CAD build for the part. Positions are in the model's coordinates, mm. A direction names the side the tool comes from. Coordinates: 2 decimals unless noted, no trailing zeros. Loops run counter-clockwise (first coordinate to the right, second up) from the corner with the lowest first, then second, coordinate; pieces in that order, holes last. Notation, with made-up numbers: (87.5, -19.5) -> (125.5, -19.5) arc R27 cw to (125.5, 13.5) -> close; hole circle Ø11 at (-28.75, 18). An arc over 180 degrees is marked (long way). Write each question's results on one line, items separated by ' | '.
```python
from build123d import *

# Parameters (mm, degrees)
SKETCH3_R                = 15
CUT_EXTRUDE1_DEPTH       = 10
SKETCH4_W                = 17
SKETCH4_H                = 15
CUT_EXTRUDE2_DEPTH       = 32.819805153
SKETCH4_4_W              = 27
SKETCH4_4_H              = 25
SKETCH4_4_W_2            = 17
SKETCH4_4_H_2            = 15
EXTRUDE_THIN2_DEPTH      = 160
SKETCH5_W                = 10
SKETCH5_H                = 60
BOSS_EXTRUDE1_DEPTH      = 3
FILLET1_R                = 4
BOSS_EXTRUDE5_DEPTH      = 9
BOSS_EXTRUDE5_DEPTH_BACK = 5
SKETCH6_W                = 36
SKETCH6_H                = 40
CUT_EXTRUDE4_DEPTH       = 17
CUT_EXTRUDE4_DEPTH_BACK  = 160
SKETCH2_3_R              = 14.5
CUT_EXTRUDE5_DEPTH       = 170.068033643
CUT_EXTRUDE5_DEPTH_BACK  = 170.068033643
SKETCH8_W                = 9
SKETCH8_H                = 8
FILLET2_R                = 34
FILLET3_R                = 34
BOSS_EXTRUDE6_DEPTH      = 20


with BuildPart() as part:
    # Extrude-Thin1: read off the stored shape, not the designer's step
    # Extrude-Thin1 outline → Extrude-Thin1 (revolve)
    with BuildSketch(Plane.XZ):
        Polygon((17.5, 20), (0, 20), (0, 17), (14.5, 17), (14.5, 3), (0, 3), (0, 0), (17.5, 0), align=None)
    revolve(axis=Axis((0, 0, 0), (0, 0, 1)))

    # Sketch3 → Cut-Extrude1 (cut)
    with BuildSketch(Plane(origin=(0, 0, 0), x_dir=(-1, 0, 0), z_dir=(0, 0, -1))):
        Circle(SKETCH3_R)
    extrude(amount=-CUT_EXTRUDE1_DEPTH, mode=Mode.SUBTRACT)

    # Sketch4 → Cut-Extrude2 (cut, through all)
    with BuildSketch(Plane(origin=(0, 0, 0), x_dir=(0, 0, -1), z_dir=(1, 0, 0))):
        with Locations((-8.5, 0)):
            Rectangle(SKETCH4_W, SKETCH4_H)
    extrude(amount=CUT_EXTRUDE2_DEPTH, mode=Mode.SUBTRACT)

    # Sketch4<4> → Extrude-Thin2 (add)
    with BuildSketch(Plane(origin=(0, 0, 0), x_dir=(0, 0, -1), z_dir=(1, 0, 0))):
        with Locations((-8.5, 0)):
            Rectangle(SKETCH4_4_W, SKETCH4_4_H)
        with Locations((-8.5, 0)):
            Rectangle(SKETCH4_4_W_2, SKETCH4_4_H_2, mode=Mode.SUBTRACT)
    extrude(amount=EXTRUDE_THIN2_DEPTH)

    # Sketch5 → Boss-Extrude1 (add)
    with BuildSketch(Plane(origin=(0, 0, 0), x_dir=(-1, 0, 0), z_dir=(0, 0, -1))):
        Rectangle(SKETCH5_W, SKETCH5_H)
    extrude(amount=-BOSS_EXTRUDE1_DEPTH)

    # Fillet1
    fillet1_edges = [part.edges().sort_by_distance(p)[0] for p in [
        (-5, 30, 1.5),
        (5, -30, 1.5),
        (-5, -30, 1.5),
        (5, 30, 1.5),
    ]]
    fillet(fillet1_edges, radius=FILLET1_R)

    # Sketch6 → Boss-Extrude5 (add, two sides: drawn at the far end of the back side and taken through both)
    with BuildSketch(Plane.ZY.offset(17.5).offset(-BOSS_EXTRUDE5_DEPTH_BACK)):
        with Locations((2, 0)):
            Rectangle(SKETCH6_W, SKETCH6_H)
    extrude(amount=BOSS_EXTRUDE5_DEPTH + BOSS_EXTRUDE5_DEPTH_BACK)

    # Sketch2<3> → Cut-Extrude4 (cut, two sides: drawn at the far end of the back side and taken through both)
    with BuildSketch(Plane.XY.offset(-CUT_EXTRUDE4_DEPTH_BACK)):
        with Locations(Location((0, 0, 0), (0, 0, 149.549685979))):
            Circle(SKETCH2_3_R)
    extrude(amount=CUT_EXTRUDE4_DEPTH + CUT_EXTRUDE4_DEPTH_BACK, mode=Mode.SUBTRACT)

    # Sketch8 → Cut-Extrude5 (cut, two sides: drawn at the far end of the back side and taken through both)
    with BuildSketch(Plane.XZ.offset(20).offset(-CUT_EXTRUDE5_DEPTH_BACK)):
        with Locations((-17, -4)):
            Rectangle(SKETCH8_W, SKETCH8_H)
    extrude(amount=CUT_EXTRUDE5_DEPTH + CUT_EXTRUDE5_DEPTH_BACK, mode=Mode.SUBTRACT)

    # Fillet2
    # the kernel refuses this fillet: 34 mm, written as the material it adds along each edge
    with BuildSketch(Plane(origin=(-12.5, -12.247448714, 0), x_dir=(0.923034160497627, -0.3847179987399096, 0), z_dir=(0, 0, 1))) as fillet2_piece_1:
        with BuildLine():
            CenterArc((26.914388587, -31.306789136), FILLET2_R, 112.958457005, 21.780491129)
            Line((2.982546016, -7.155869668), (2.503909164, -6.672851279))
            ThreePointArc((2.503909164, -6.672851279), (0.863609779, -3.839543073), (-0.627663229, -0.261608239))
            Line((-0.627663229, -0.261608239), (0.26524325, 0.626135783))
            ThreePointArc((0.26524325, 0.626135783), (6.826113047, -0.706211474), (13.386982845, 0.626135783))
            Line((13.386982845, 0.626135783), (13.652226095, 0))
        make_face()
    extrude(amount=20)
    with BuildSketch(Plane(origin=(-12.5, 12.247448714, 0), x_dir=(0, 1, 0), z_dir=(0, 0, 1))) as fillet2_piece_2:
        with BuildLine():
            CenterArc((39.251685543, -12.798614811), FILLET2_R, 157.887286265, 21.780491129)
            Line((5.252257101, -12.601471052), (4.572268533, -12.597528177))
            ThreePointArc((4.572268533, -12.597528177), (3.277985866, -6.029043261), (-0.475900864, -0.485714286))
            Line((-0.475900864, -0.485714286), (0, 0.68))
            ThreePointArc((0, 0.68), (3.876275643, 0.68), (7.122568601, 0.255972296))
            Line((7.122568601, 0.255972296), (7.752551286, 0))
        make_face()
    extrude(amount=20)

    # Fillet3
    # the kernel refuses this fillet: 34 mm, written as the material it adds along each edge
    with BuildSketch(Plane(origin=(0, 12.5, 20), x_dir=(-1, 0, 0), z_dir=(0, -1, 0))) as fillet3_piece_1:
        with BuildLine():
            CenterArc((11.489125293, -34), FILLET3_R, 90, 19.749922796)
            Line((0, -2), (0, 0))
            Line((0, 0), (11.489125293, 0))
        make_face()
    extrude(amount=25)

    # Sketch9 → Boss-Extrude6 (add)
    with BuildSketch(Plane.XY.offset(22)):
        with BuildLine():
            Line((136.437253933, 1), (134.437253933, 1))
            Line((134.437253933, 1), (134.437253933, -1))
            Line((134.437253933, -1), (136.437253933, -1))
            ThreePointArc((136.437253933, -1), (135.89103626, -3.061467459), (134.819592861, -4.905379299))
            Line((134.819592861, -4.905379299), (133.405379299, -3.491165737))
            Line((133.405379299, -3.491165737), (131.991165737, -4.905379299))
            Line((131.991165737, -4.905379299), (133.405379299, -6.319592861))
            ThreePointArc((133.405379299, -6.319592861), (131.561467459, -7.39103626), (129.5, -7.937253933))
            Line((129.5, -7.937253933), (129.5, -5.937253933))
            Line((129.5, -5.937253933), (127.5, -5.937253933))
            Line((127.5, -5.937253933), (127.5, -7.937253933))
            ThreePointArc((127.5, -7.937253933), (125.438532541, -7.39103626), (123.594620701, -6.319592861))
            Line((123.594620701, -6.319592861), (125.008834263, -4.905379299))
            Line((125.008834263, -4.905379299), (123.594620701, -3.491165737))
            Line((123.594620701, -3.491165737), (122.180407139, -4.905379299))
            ThreePointArc((122.180407139, -4.905379299), (121.10896374, -3.061467459), (120.562746067, -1))
            Line((120.562746067, -1), (122.562746067, -1))
            Line((122.562746067, -1), (122.562746067, 1))
            Line((122.562746067, 1), (120.562746067, 1))
            ThreePointArc((120.562746067, 1), (121.10896374, 3.061467459), (122.180407139, 4.905379299))
            Line((122.180407139, 4.905379299), (123.594620701, 3.491165737))
            Line((123.594620701, 3.491165737), (125.008834263, 4.905379299))
            Line((125.008834263, 4.905379299), (123.594620701, 6.319592861))
            ThreePointArc((123.594620701, 6.319592861), (125.438532541, 7.39103626), (127.5, 7.937253933))
            Line((127.5, 7.937253933), (127.5, 5.937253933))
            Line((127.5, 5.937253933), (129.5, 5.937253933))
            Line((129.5, 5.937253933), (129.5, 7.937253933))
            ThreePointArc((129.5, 7.937253933), (131.561467459, 7.39103626), (133.405379299, 6.319592861))
            Line((133.405379299, 6.319592861), (131.991165737, 4.905379299))
            Line((131.991165737, 4.905379299), (133.405379299, 3.491165737))
            Line((133.405379299, 3.491165737), (134.819592861, 4.905379299))
            ThreePointArc((134.819592861, 4.905379299), (135.89103626, 3.061467459), (136.437253933, 1))
        make_face()
    extrude(amount=BOSS_EXTRUDE6_DEPTH)


solid = part.part
```
Q1. Which spindle directions (+Z, -Z, +X, -X, +Y, -Y) get a long thin tool onto all of the face, cutting with end or side? Do faces 1 (the cylindrical face through (121.098, 3.034, 31.86)), 2 (the cylindrical face through (125.466, -7.402, 31.86)), 3 (the cylindrical face through (135.88, 3.09, 31.86)). Say none if no direction does.
Results are:
face 1: +Z, -X, +Y | face 2: +Z, -X, -Y | face 3: +Z, +X, +Y
Q2. Drop flat-ended pins along their axis: pin 1 (1.6 mm diameter, centred on y = 7, z = 34.5, fed in from -X); pin 2 (1 mm diameter, centred on x = 134, z = 28, fed in from -Y); pin 3 (8.5 mm diameter, centred on x = 66.5, z = 10.5, fed in from +Y). Give the stop position or say it passes through.
Results are:
pin 1: x = 123.59 | pin 2: y = -4.59 | pin 3: y = 12.5
Q3. Cut at A-A on x = 58.5. Write the cut outline in (y, z), and give its area (3 significant figures).
Results are:
outline: (-12.5, -5) -> (12.5, -5) -> (12.5, 22) -> (-12.5, 22) -> close; hole (-7.5, 0) -> (7.5, 0) -> (7.5, 17) -> (-7.5, 17) -> close | area: 420 mm^2
Q4. Wall check: L1, parallel to Z at x = 32.5, y = 3; L2, parallel to Y at x = 0, z = 11; L3, parallel to Y at x = 119.5, z = 5. Give the ranges that are in metal, low to high. Write a range as from..to.
Results are:
L1: -5..0, 17..22 | L2: -17.5..-14.5, 14.5..17.5 | L3: -12.5..-7.5, 7.5..12.5
Q5. Pull direction X, two halves, no side cores. Call faces 4 (the flat face through (-3.6, -14.3, 10)), 5 (the cylindrical face through (125.41, 7.38, 31.86)), 6 (the cylindrical face through (3.859, -28.797, 1.521)), 7 (the cylindrical face through (10.61, -9.883, 8.29)): +X half, -X half, draft (parallel to the pull), parting line (faces both ways), or undercut.
Results are:
face 4: undercut | face 5: -X half | face 6: +X half | face 7: undercut
